Design review of the part built by this model. Coordinates are the model's own, in mm. A direction names the side the tool comes from. Coordinates: 2 decimals unless noted, no trailing zeros. Write each loop counter-clockwise with the first axis right and the second up, starting at its lowest first coordinate (ties: lowest second). Pieces come first, ordered by that corner, then holes.
Q1. Mouldability with a two-part tool opening along Y and no side actions: class faces 6 (the flat face through (24, 10, 11)), 7 (the cylindrical face through (77.675, 2.24, 6.983)), 8 (the flat face through (30, 17.1, 14)) as pulls with the +Y half, pulls with the -Y half, needs draft (parallel to the pull), parting line crosses it, or undercut.
Q2. Machinability: for faces 1 (the cylindrical face through (32.15, 6.38, 34.82)), 2 (the flat face through (60, 5, 27)), 3 (the flat face through (20, 3, 5)), 4 (the cylindrical face through (30.25, 9.98, 35.14)), 5 (the cylindrical face through (31.595, 14.079, 37.955)), which of the approach directions +Z, -Z, +X, -X, +Y, -Y give a long, thin tool a straight path to every point of the face, cutting with its end or side? Answer none if there is none.
Q3. Insertion check: pin 1 (2 mm diameter, centred on x = 80.5, y = 30.5, fed in from +Z); pin 2 (2.5 mm diameter, centred on x = 28, z = 35.5, fed in from -Y); pin 3 (4 mm diameter, centred on y = 10.35, z = 13, fed in from -X); pin 4 (2.5 mm diameter, centred on y = 2.5, z = 5, fed in from -X). Each pin has a flat end and moves straight along its axis. Give the tip position at first contact, or say it passes through.
Q4. Take a section at A-A (x = 85). Give the boundary of the cut face in (y, z).
Q5. Take a section at B-B (y = 25). Give the boundary of the cut face in (x, z).
Q6. For probe 1 along Y at (x, z) = (53, 1.5); probe 2 along Z at (x, y) = (70.5, 2.5); probe 3 along X at (y, z) = (8, 24), list the stretches that pass through material, from the lowest coordinate up.
```python
from build123d import *

# Parameters (mm, degrees)
F0_W      = 90
F0_H      = 70
F0_R      = 1.7
F0_R_2    = 1.75
F1_DEPTH  = 5
F2_W      = 90
F2_H      = 5
F3_DEPTH  = 45
F4_W      = 11
F4_H      = 45
F5_DEPTH  = 12.1
F6_R      = 6.25
F7_DEPTH  = 25
F8_R      = 8.15
F9_DEPTH  = 5
F10_R     = 10
F11_DEPTH = 5
F12_R     = 8.15
F13_DEPTH = 2.8
F14_R     = 1.6
F14_R_2   = 11.25
F15_DEPTH = 25
F17_DEPTH = 4
F19_DEPTH = 4
F20_R     = 4
F21_DEPTH = 5
F22_R     = 2
F23_DEPTH = 20
F24_SIZE  = 1
F26_R     = 2.25
F28_R     = 2
F29_DEPTH = 25


with BuildPart() as f1:
    # F0 (on Top) → F1 (new body)
    with BuildSketch(Plane.XY):
        with Locations((45, 35)):
            Rectangle(F0_W, F0_H)
        with Locations((35, 25)):
            Circle(F0_R, mode=Mode.SUBTRACT)
        with Locations((55, 25)):
            Circle(F0_R, mode=Mode.SUBTRACT)
        with Locations((35, 45)):
            Circle(F0_R, mode=Mode.SUBTRACT)
        with Locations((5, 61.554949)):
            Circle(F0_R_2, mode=Mode.SUBTRACT)
        with Locations((5, 66.554949)):
            Circle(F0_R_2, mode=Mode.SUBTRACT)
        with Locations((21, 61.554949)):
            Circle(F0_R_2, mode=Mode.SUBTRACT)
        with Locations((21, 66.554949)):
            Circle(F0_R_2, mode=Mode.SUBTRACT)
        with Locations((37, 61.554949)):
            Circle(F0_R_2, mode=Mode.SUBTRACT)
        with Locations((37, 66.554949)):
            Circle(F0_R_2, mode=Mode.SUBTRACT)
        with Locations((55, 45)):
            Circle(F0_R, mode=Mode.SUBTRACT)
        with Locations((53, 61.554949)):
            Circle(F0_R_2, mode=Mode.SUBTRACT)
        with Locations((53, 66.554949)):
            Circle(F0_R_2, mode=Mode.SUBTRACT)
        with Locations((69, 61.554949)):
            Circle(F0_R_2, mode=Mode.SUBTRACT)
        with Locations((69, 66.554949)):
            Circle(F0_R_2, mode=Mode.SUBTRACT)
        with Locations((85, 61.554949)):
            Circle(F0_R_2, mode=Mode.SUBTRACT)
        with Locations((85, 66.554949)):
            Circle(F0_R_2, mode=Mode.SUBTRACT)
    extrude(amount=F1_DEPTH)

    # F2 (on face) → F3 (join)
    with BuildSketch(Plane.XY.offset(5)):
        with Locations((45, 2.5)):
            Rectangle(F2_W, F2_H)
    extrude(amount=F3_DEPTH)

    # F4 (on face) → F5 (join)
    with BuildSketch(Plane(origin=(0, 5, 0), x_dir=(-1, 0, 0), z_dir=(0, 1, 0))):
        with Locations((-29.5, 27.5)):
            Rectangle(F4_W, F4_H)
    extrude(amount=F5_DEPTH)

    # F6 (on face) → F7 (cut)
    with BuildSketch(Plane(origin=(0, 17.1, 0), x_dir=(-1, 0, 0), z_dir=(0, 1, 0))):
        with Locations((-24, 35)):
            Circle(F6_R)
    extrude(amount=-F7_DEPTH, mode=Mode.SUBTRACT)

    # F8 (on face) → F9 (cut)
    with BuildSketch(Plane(origin=(0, 17.1, 0), x_dir=(-1, 0, 0), z_dir=(0, 1, 0))):
        with Locations((-24, 35)):
            Circle(F8_R)
    extrude(amount=-F9_DEPTH, mode=Mode.SUBTRACT)

    # F10 (on face) → F11 (cut)
    with BuildSketch(Plane.XZ):
        with Locations((22.587966, 34.833703)):
            Circle(F10_R)
    extrude(amount=-F11_DEPTH, mode=Mode.SUBTRACT)

    # F12 (on face) → F13 (cut)
    with BuildSketch(Plane.XZ.offset(-5)):
        with Locations((24, 35)):
            Circle(F12_R)
    extrude(amount=-F13_DEPTH, mode=Mode.SUBTRACT)

    # F14 (on face) → F15 (cut)
    with BuildSketch(Plane(origin=(24, 0, 0), x_dir=(0, -1, 0), z_dir=(-1, 0, 0))):
        with Locations((-10.35, 44.5)):
            Circle(F14_R)
        with Locations((-10.35, 13)):
            Circle(F14_R)
        with Locations((-26.1, 28.75)):
            Circle(F14_R_2)
    extrude(amount=-F15_DEPTH, mode=Mode.SUBTRACT)

    # F16 (on face) → F17 (join)
    with BuildSketch(Plane(origin=(0, 0, 0), x_dir=(0, -1, 0), z_dir=(-1, 0, 0))):
        Polygon((0, 50), (-5, 50), (-55, 5), (-55, 0), (0, 0), align=None)
    extrude(amount=-F17_DEPTH)

    # F18 (on face) → F19 (join)
    with BuildSketch(Plane.YZ.offset(90)):
        Polygon((55, 5), (5, 50), (0, 50), (0, 0), (55, 0), align=None)
    extrude(amount=-F19_DEPTH)

    # F20 (on face) → F21 (cut)
    with BuildSketch(Plane(origin=(0, 0, 0), x_dir=(0, -1, 0), z_dir=(-1, 0, 0))):
        with Locations((-10.391034, 44.5)):
            Circle(F20_R)
        with Locations((-10.391034, 13)):
            Circle(F20_R)
    extrude(amount=-F21_DEPTH, mode=Mode.SUBTRACT)

    # F22 (on face) → F23 (cut)
    with BuildSketch(Plane(origin=(0, 0, 0), x_dir=(0, -1, 0), z_dir=(-1, 0, 0))):
        with Locations((-2.5, 5)):
            Circle(F22_R)
        with Locations((-2.5, 30)):
            Circle(F22_R)
    extrude(amount=-F23_DEPTH, mode=Mode.SUBTRACT)

    # F24
    f24_edges = [f1.edges().sort_by_distance(p)[0] for p in [
        (33.3, 45, 5),
        (53.3, 45, 5),
        (53.3, 25, 5),
        (33.3, 25, 5),
    ]]
    chamfer(f24_edges, length=F24_SIZE)

    # F27: sweep along a path in F25
    with BuildLine(Plane(origin=(24, 0, 0), x_dir=(0, -1, 0), z_dir=(-1, 0, 0))) as f27_path:
        Line((1.5, 28.5), (-22.1, 8.5))
    # F26 (on face) → F27 (sweep, cut)
    with BuildSketch(Plane.XZ):
        with Locations((23.989582, 28.05)):
            Circle(F26_R)
    sweep(path=f27_path.line, mode=Mode.SUBTRACT)

    # F28 (on face) → F29 (cut)
    with BuildSketch(Plane.YZ.offset(90)):
        with Locations((2.5, 5)):
            Circle(F28_R)
        with Locations((2.5, 30)):
            Circle(F28_R)
    extrude(amount=-F29_DEPTH, mode=Mode.SUBTRACT)


solid = f1.part
```
Response:
1. face 6: needs draft
1. face 7: undercut
1. face 8: pulls with the +Y half
2. face 1: -Y
2. face 2: +Z, +Y
2. face 3: -X
2. face 4: +Y, -Y
2. face 5: +Y
3. pin 1: stops at z = 5
3. pin 2: passes through
3. pin 3: stops at x = 24
3. pin 4: stops at x = 20
4. outline: (0, 0) - (59.8, 0) - (59.8, 5) - (5, 5) - (5, 50) - (0, 50) - close; (63.3, 0) - (64.8, 0) - (64.8, 5) - (63.3, 5) - close; (68.3, 0) - (70, 0) - (70, 5) - (68.3, 5) - close; hole circle Ø4 at (2.5, 5); hole circle Ø4 at (2.5, 30)
5. outline: (0, 0) - (33.3, 0) - (33.3, 4) - (32.3, 5) - (4, 5) - (4, 32) - (0, 32) - close; (36.7, 0) - (53.3, 0) - (53.3, 4) - (52.3, 5) - (37.7, 5) - (36.7, 4) - close; (56.7, 0) - (90, 0) - (90, 32) - (86, 32) - (86, 5) - (57.7, 5) - (56.7, 4) - close
6. probe 1: y = 0 to 59.8, 63.3 to 64.8, 68.3 to 70
6. probe 2: z = 0 to 3, 7 to 28, 32 to 50
6. probe 3: x = 0 to 4, 24 to 35, 86 to 90
